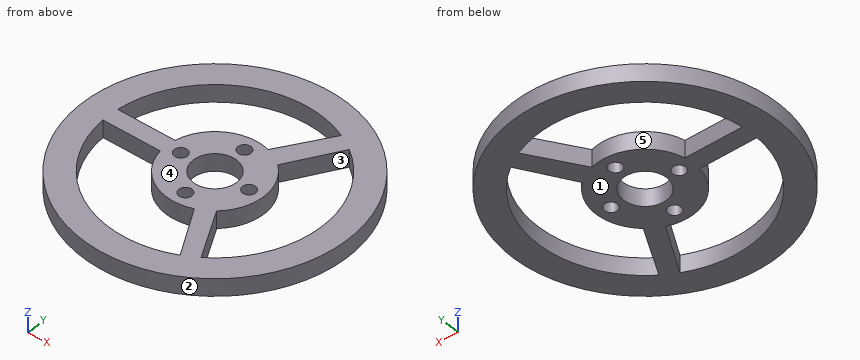
```python
from build123d import *

# Parameters (mm, degrees)
SKETCH_1_R          = 30.5
EXTRUDE_1_DEPTH     = 4
CUT_EXTRUDE_1_REACH = 6
SKETCH_2_R          = 5
SKETCH_2_R_2        = 1.5


with BuildPart() as part:
    # 草图1 → 凸台-拉伸1 (new body)
    with BuildSketch(Plane.XY):
        Circle(SKETCH_1_R)
    extrude(amount=EXTRUDE_1_DEPTH)

    # 草图2 → 切除-拉伸1 (cut, up to next)
    with BuildSketch(Plane.XY.offset(4), mode=Mode.PRIVATE) as cut_extrude_1_sk1:
        Circle(SKETCH_2_R)
    cut_extrude_1_tool1 = extrude(cut_extrude_1_sk1.sketch, amount=-CUT_EXTRUDE_1_REACH, mode=Mode.PRIVATE) & part.part
    add(cut_extrude_1_tool1.solids().sort_by_distance((0, 0, 4))[0], mode=Mode.SUBTRACT)
    # 草图2 → 切除-拉伸1 (cut, up to next)
    with BuildSketch(Plane.XY.offset(4), mode=Mode.PRIVATE) as cut_extrude_1_sk2:
        with Locations((-8, 0)):
            Circle(SKETCH_2_R_2)
    cut_extrude_1_tool2 = extrude(cut_extrude_1_sk2.sketch, amount=-CUT_EXTRUDE_1_REACH, mode=Mode.PRIVATE) & part.part
    add(cut_extrude_1_tool2.solids().sort_by_distance((-8, 0, 4))[0], mode=Mode.SUBTRACT)
    # 草图2 → 切除-拉伸1 (cut, up to next)
    with BuildSketch(Plane.XY.offset(4), mode=Mode.PRIVATE) as cut_extrude_1_sk3:
        with Locations((0, 8)):
            Circle(SKETCH_2_R_2)
    cut_extrude_1_tool3 = extrude(cut_extrude_1_sk3.sketch, amount=-CUT_EXTRUDE_1_REACH, mode=Mode.PRIVATE) & part.part
    add(cut_extrude_1_tool3.solids().sort_by_distance((0, 8, 4))[0], mode=Mode.SUBTRACT)
    # 草图2 → 切除-拉伸1 (cut, up to next)
    with BuildSketch(Plane.XY.offset(4), mode=Mode.PRIVATE) as cut_extrude_1_sk4:
        with Locations((8, 0)):
            Circle(SKETCH_2_R_2)
    cut_extrude_1_tool4 = extrude(cut_extrude_1_sk4.sketch, amount=-CUT_EXTRUDE_1_REACH, mode=Mode.PRIVATE) & part.part
    add(cut_extrude_1_tool4.solids().sort_by_distance((8, 0, 4))[0], mode=Mode.SUBTRACT)
    # 草图2 → 切除-拉伸1 (cut, up to next)
    with BuildSketch(Plane.XY.offset(4), mode=Mode.PRIVATE) as cut_extrude_1_sk5:
        with Locations((0, -8)):
            Circle(SKETCH_2_R_2)
    cut_extrude_1_tool5 = extrude(cut_extrude_1_sk5.sketch, amount=-CUT_EXTRUDE_1_REACH, mode=Mode.PRIVATE) & part.part
    add(cut_extrude_1_tool5.solids().sort_by_distance((0, -8, 4))[0], mode=Mode.SUBTRACT)
    # 草图2 → 切除-拉伸1 (cut, up to next)
    with BuildSketch(Plane.XY.offset(4), mode=Mode.PRIVATE) as cut_extrude_1_sk6:
        with BuildLine():
            Line((-24.519245453, -2), (-11.082272055, -2))
            ThreePointArc((-11.082272055, -2), (-5.44406657, -9.857935539), (4.209531065, -10.444931887))
            Line((4.209531065, -10.444931887), (10.909403583, -22.049451491))
            ThreePointArc((10.909403583, -22.049451491), (-12.116190623, -21.410075254), (-24.519245453, -2))
        make_face()
    cut_extrude_1_tool6 = extrude(cut_extrude_1_sk6.sketch, amount=-CUT_EXTRUDE_1_REACH, mode=Mode.PRIVATE) & part.part
    add(cut_extrude_1_tool6.solids().sort_by_distance((-7.903429, -14.053546, 4))[0], mode=Mode.SUBTRACT)
    # 草图2 → 切除-拉伸1 (cut, up to next)
    with BuildSketch(Plane.XY.offset(4), mode=Mode.PRIVATE) as cut_extrude_1_sk7:
        with BuildLine():
            Line((-24.519245453, 2), (-11.082272055, 2))
            ThreePointArc((-11.082272055, 2), (-5.942459521, 9.565768592), (3.117477103, 10.821187108))
            Line((3.117477103, 10.821187108), (10.304921695, 22.338352367))
            ThreePointArc((10.304921695, 22.338352367), (-12.406606878, 21.243104843), (-24.519245453, 2))
        make_face()
    cut_extrude_1_tool7 = extrude(cut_extrude_1_sk7.sketch, amount=-CUT_EXTRUDE_1_REACH, mode=Mode.PRIVATE) & part.part
    add(cut_extrude_1_tool7.solids().sort_by_distance((-8.308104, 14.002241, 4))[0], mode=Mode.SUBTRACT)
    # 草图2 → 切除-拉伸1 (cut, up to next)
    with BuildSketch(Plane.XY.offset(4), mode=Mode.PRIVATE) as cut_extrude_1_sk8:
        with BuildLine():
            Line((14.155543142, -20.119989959), (7.597126799, -8.312666138))
            ThreePointArc((7.597126799, -8.312666138), (11.258684205, 0.242453893), (7.232225933, 8.632013784))
            Line((7.232225933, 8.632013784), (13.976038331, 20.245092002))
            ThreePointArc((13.976038331, 20.245092002), (24.600435555, 0.109398924), (14.155543142, -20.119989959))
        make_face()
    cut_extrude_1_tool8 = extrude(cut_extrude_1_sk8.sketch, amount=-CUT_EXTRUDE_1_REACH, mode=Mode.PRIVATE) & part.part
    add(cut_extrude_1_tool8.solids().sort_by_distance((16.242658, 0.143003, 4))[0], mode=Mode.SUBTRACT)


solid = part.part
```
Model file for the job. Use its own axes, mm. Face numbers are marked on the shaded views. A direction names the side the tool comes from. Give positions to 0.01 mm unless a question says otherwise; leave off trailing zeros. Order: outer loops, then holes, each group sorted by start corner. A loop starts at its lowest first (then second) coordinate and runs counter-clockwise, first axis right, second up.
1) Saw through at A-A, the plane z = 0.85. Count the separate pieces of the cut face and the enclosed holes in it, then the cut area to 3 significant figures.
2) 3-axis set-ups, long thin cutter, end or side, ignore diameter. For the marked faces 4 and 5: which of +Z, -Z, +X, -X, +Y, -Y reach the whole face in a straight line?
3) Saw through at B-B, the plane y = 0. Write the cut outline in (x, z).
4) Mould opens along X. For the marked faces 1, 2 and 3 say: +X half, -X half, draft (parallel to the pull), parting line (faces both ways), or undercut.
5) Saw through at D-D, the plane y = 16. Write the cut outline in (x, z), then the cut area to 3 significant figures.
6) Saw through at C-C, the plane x = 20. Write the cut outline in (y, z), then the cut area to 3 significant figures.
7) Pin check, flat tips, straight feed: pin 1 (2 mm diameter, centred on x = -16.5, z = 2, fed in from +Y); pin 2 (1 mm diameter, centred on y = 4.5, z = 2, fed in from -X). Stop position of each tip, or through.
8) Wall check: probe 1 along Y at (x, z) = (0, 3.05); probe 2 along X at (y, z) = (7, 0.8); probe 3 along X at (y, z) = (-17, 2). Give the ranges that are in metal, low to high.
Computed:
1. separate pieces: 1
1. enclosed holes: 8
1. area: 1,480 mm2
2. face 4: +Z, +X, -X, +Y, -Y
2. face 5: +Z, -Z
3. outline: (-30.5, 0) - (-9.5, 0) - (-9.5, 4) - (-30.5, 4) - close; (-6.5, 0) - (-5, 0) - (-5, 4) - (-6.5, 4) - close; (5, 0) - (6.5, 0) - (6.5, 4) - (5, 4) - close; (9.5, 0) - (11.26, 0) - (11.26, 4) - (9.5, 4) - close; (24.6, 0) - (30.5, 0) - (30.5, 4) - (24.6, 4) - close
4. face 1: draft
4. face 2: parting line
4. face 3: undercut
5. outline: (-25.97, 0) - (-18.69, 0) - (-18.69, 4) - (-25.97, 4) - close; (6.35, 0) - (11.51, 0) - (11.51, 4) - (6.35, 4) - close; (18.69, 0) - (25.97, 0) - (25.97, 4) - (18.69, 4) - close
5. area: 78.9 mm2
6. outline: (-23.03, 0) - (-14.32, 0) - (-14.32, 4) - (-23.03, 4) - close; (14.32, 0) - (23.03, 0) - (23.03, 4) - (14.32, 4) - close
6. area: 69.6 mm2
7. pin 1: stops at y = 26.27
7. pin 2: stops at x = -30.24
8. probe 1: y = -30.5 to -24.6, -11.26 to -9.5, -6.5 to -5, 5 to 6.5, 9.5 to 11.26, 24.6 to 30.5
8. probe 2: x = -29.69 to -23.58, -8.82 to -1.12, 1.12 to 8.82, 23.58 to 29.69
8. probe 3: x = -25.32 to -17.78, 7.99 to 12.42, 17.78 to 25.32
